Model file for the job. Use its own axes, mm. A direction names the side the tool comes from. Coordinates: 2 decimals unless noted, no trailing zeros. Order: outer loops, then holes, each group sorted by start corner. A loop starts at its lowest first (then second) coordinate and runs counter-clockwise, first axis right, second up.
from build123d import *

# Parameters (mm, degrees)
CUT_EXTRUDE1_DEPTH = 5.1


with BuildPart() as part:
    # Sketch1 → Revolve1 (revolve)
    with BuildSketch(Plane(origin=(0, 0, 0), x_dir=(0, 0, -1), z_dir=(1, 0, 0))):
        with BuildLine():
            Line((0, 0), (0, 5.9))
            Line((0, 5.9), (7.417157288, 5.9))
            Line((7.417157288, 5.9), (7.7, 5.617157288))
            Line((7.7, 5.617157288), (7.7, 4.9))
            Line((7.7, 4.9), (10.1, 4.9))
            Line((10.1, 4.9), (10.2, 4.8))
            Line((10.2, 4.8), (10.3, 4.9))
            Line((10.3, 4.9), (11, 4.9))
            Line((11, 4.9), (11.2, 4.7))
            Line((11.2, 4.7), (11.2, 3.875))
            Line((11.2, 3.875), (11.725, 3.875))
            ThreePointArc((11.725, 3.875), (11.990165043, 3.984834957), (12.1, 4.25))
            Line((12.1, 4.25), (12.1, 5.9))
            Line((12.1, 5.9), (13.504587146, 5.9))
            ThreePointArc((13.504587146, 5.9), (13.633144667, 5.853208889), (13.701548696, 5.734729636))
            Line((13.701548696, 5.734729636), (14.1, 3.475))
            Line((14.1, 3.475), (14.1, 0))
            Line((14.1, 0), (0, 0))
        make_face()
    revolve(axis=Axis((0, 0, -14.1), (0, 0, 1)))

    # Sketch2 → Revolve2 (revolve)
    with BuildSketch(Plane(origin=(0, 0, 0), x_dir=(0, 0, -1), z_dir=(1, 0, 0))):
        Polygon((-8, 0), (-8, 4.158121832), (-6.93615215, 4.772334675), (0, 4.988878168), (0, 0), align=None)
    revolve(axis=Axis((0, 0, 0), (0, 0, 1)))

    # Sketch3 → Cut-Revolve1 (revolve, cut)
    with BuildSketch(Plane(origin=(0, 0, 0), x_dir=(0, 0, -1), z_dir=(1, 0, 0))):
        Polygon((0, 5.9), (0, 5), (1.3, 5), (1.3, 5.7), (1.5, 5.9), align=None)
    revolve(axis=Axis((0, 0, -50), (0, 0, 1)), mode=Mode.SUBTRACT)

    # Sketch4 → Cut-Revolve2 (revolve, cut)
    with BuildSketch(Plane(origin=(0, 0, 0), x_dir=(0, 0, -1), z_dir=(1, 0, 0))):
        with BuildLine():
            Line((-8, 0), (-8, 2.6))
            Line((-8, 2.6), (-7.5, 2.1))
            Line((-7.5, 2.1), (-2.9, 2.1))
            Line((-2.9, 2.1), (-2.9, 3.175))
            Line((-2.9, 3.175), (13.8, 3.175))
            ThreePointArc((13.8, 3.175), (14.012132034, 3.262867966), (14.1, 3.475))
            Line((14.1, 3.475), (14.1, 0))
            Line((14.1, 0), (-8, 0))
        make_face()
    revolve(axis=Axis((0, 0, -14.1), (0, 0, 1)), mode=Mode.SUBTRACT)

    # Sketch5 → Cut-Extrude1 (cut)
    with BuildSketch(Plane.XY.offset(2.9)):
        Polygon((-2, -1.154700538), (0, -2.309401077), (2, -1.154700538), (2, 1.154700538), (0, 2.309401077), (-2, 1.154700538), align=None)
    extrude(amount=CUT_EXTRUDE1_DEPTH, mode=Mode.SUBTRACT)


solid = part.part
Q1. Which spindle directions (+Z, -Z, +X, -X, +Y, -Y) get a long thin tool onto all of the face, cutting with end or side? Do faces 1 (the face through (4.766, -1.058, 3.42)), 2 (the face through (-2.1, 0, 5.2)), 3 (the face through (4.783, -1.062, -10.655)), 4 (the face through (3.1, -0.69, -5.57)). Say none if no direction does.
Established:
face 1: +Z
face 2: +Z, -Z
face 3: none
face 4: -Z
Q2. Probe line 1 (Y direction, x = 0, z = -7.75) (3 decimals); line 2 (X direction, y = 0, z = -3.25) (3 decimals). List the from-to ranges inside material, lowest first.
Established:
line 1: y = -4.9 to -3.175, 3.175 to 4.9
line 2: x = -5.9 to -3.175, 3.175 to 5.9
Q3. Drop flat-ended pins along their axis: P1, Ø1.9, axis at x = 0, y = 1.5, coming from the -Z side; P2, Ø3, axis at x = 3.5, z = 4.5, coming from the +Y side; P3, Ø2, axis at x = 3, z = -3, coming from the +Y side. Give the stop position or say it passes through.
Established:
P1: stops at z = 2.9
P2: stops at y = 4.42
P3: stops at y = 5.55
Q4. Cut at A-A, the plane z = -0.5. List the corners of the cut face in (x, y) (3 decimals).
Established:
outline: circle Ø10 at (0, 0); hole circle Ø6.35 at (0, 0)
Q5. Mould opens along X. For faces 5 (the face through (1.058, 1.814, 5.168)), 6 (the face through (2, 2, 8)), 7 (the face through (-3.842, -0.504, -11.466)) say: pulls with the +X half, pulls with the -X half, needs draft (parallel to the pull), parting line crosses it, or undercut.
Established:
face 5: undercut
face 6: needs draft
face 7: parting line crosses it
Q6. Cut at B-B, the plane z = -8. List the corners of the cut face in (x, y) (3 decimals).
Established:
outline: circle Ø9.8 at (0, 0); hole circle Ø6.35 at (0, 0)
